```python
from build123d import *

# Parameters (mm, degrees)
SKETCH_1_W      = 33
SKETCH_1_H      = 22
EXTRUDE_1_DEPTH = 3


with BuildPart() as part:
    # 草图1 → 凸台-拉伸1 (new body)
    with BuildSketch(Plane.XY):
        Polygon((12.097999847, 68.896913641), (23.174949538, 68.896913641), (23.174949538, -21.103086359), (33.727403861, -21.103086359), (33.727403861, -81.103086359), (13.227403861, -81.103086359), (13.227403861, -107.603086359), (-25.772596139, -107.603086359), (-25.772596139, -81.103086359), (-46.272596139, -81.103086359), (-46.272596139, -21.103086359), (-36.272596139, -21.103086359), (-36.272596139, 68.896913641), (-25.195646449, 68.896913641), (-25.195646449, -21.103086359), (12.097999847, -21.103086359), align=None)
        with BuildLine():
            Line((-33.148823301, 45.73159086), (-33.148823301, 60.73159086))
            ThreePointArc((-33.148823301, 60.73159086), (-31.548823301, 62.33159086), (-29.948823301, 60.73159086))
            Line((-29.948823301, 60.73159086), (-29.948823301, 45.73159086))
            ThreePointArc((-29.948823301, 45.73159086), (-31.548823301, 44.13159086), (-33.148823301, 45.73159086))
        make_face(mode=Mode.SUBTRACT)
        with BuildLine():
            Line((20.051176699, 45.73159086), (20.051176699, 60.73159086))
            ThreePointArc((20.051176699, 60.73159086), (18.451176699, 62.33159086), (16.851176699, 60.73159086))
            Line((16.851176699, 60.73159086), (16.851176699, 45.73159086))
            ThreePointArc((16.851176699, 45.73159086), (18.451176699, 44.13159086), (20.051176699, 45.73159086))
        make_face(mode=Mode.SUBTRACT)
        with Locations((-6.272596139, -93.603086359)):
            Rectangle(SKETCH_1_W, SKETCH_1_H, mode=Mode.SUBTRACT)
    extrude(amount=EXTRUDE_1_DEPTH)


solid = part.part
```
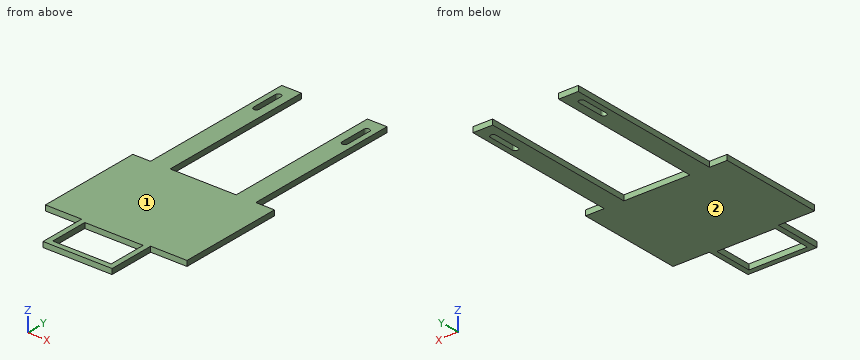
For this review, take the finished solid that the model builds, in its own axes (mm). Face numbers are marked on the shaded views. Round coordinates to 2 decimals unless told otherwise and drop trailing zeros. Write each loop counter-clockwise with the first axis right and the second up, starting at its lowest first coordinate (ties: lowest second). Pieces come first, ordered by that corner, then holes. Notation, with made-up numbers: (-21.75, -2) -> (26.25, -2) arc R8 ccw to (26.25, 8) -> close; hole circle Ø11 at (-31.75, 70.25). An arc over 180 degrees is marked (long way). One line per question, with ' | ' between items. Start each with the question number.
(1) For line 1 along Y through (x, z) = (-11.5, 2.15); line 2 along X through (y, z) = (4.5, 2.2); line 3 along X through (y, z) = (54.5, 2), list the stretches that pass through material, from the lowest coordinate up. Write a range as from..to.
(2) Add section B-B, the plane z = 0.7. Write out the cut boundary in (x, y), plus the area to 3 significant figures.
(3) Mouldability with a two-part tool opening along Z and no side actions: class the marked faces 1 and 2 as released by +Z, released by -Z, zero draft, split by the parting line, or undercut.
(4) Add section C-C, the plane x = 8. Write out the cut boundary in (y, z).
(5) Insertion check: P1, Ø0.9, axis at x = -39, z = 1, coming from the -Y side; P2, Ø0.9, axis at y = 51, z = 1, coming from the -X side; P3, Ø1.5, axis at x = -10, z = 1, coming from the +Y side. Each pin has a flat end and moves straight along its axis. Give the tip position at first contact, or say it passes through.
(6) Add section D-D, the plane x = -27.5. Write out the cut boundary in (y, z).
(7) Add section A-A, the plane y = 38. Write out the cut boundary in (x, z), plus the area to 3 significant figures.
Answer list:
1) line 1: -107.6..-104.6, -82.6..-21.1 | line 2: -36.27..-25.2, 12.1..23.17 | line 3: -36.27..-33.15, -29.95..-25.2, 12.1..16.85, 20.05..23.17
2) outline: (-46.27, -81.1) -> (-25.77, -81.1) -> (-25.77, -107.6) -> (13.23, -107.6) -> (13.23, -81.1) -> (33.73, -81.1) -> (33.73, -21.1) -> (23.17, -21.1) -> (23.17, 68.9) -> (12.1, 68.9) -> (12.1, -21.1) -> (-25.2, -21.1) -> (-25.2, 68.9) -> (-36.27, 68.9) -> (-36.27, -21.1) -> (-46.27, -21.1) -> close; hole (-33.15, 45.73) arc R1.6 ccw to (-29.95, 45.73) -> (-29.95, 60.73) arc R1.6 ccw to (-33.15, 60.73) -> close; hole (-22.77, -104.6) -> (10.23, -104.6) -> (10.23, -82.6) -> (-22.77, -82.6) -> close; hole (16.85, 45.73) arc R1.6 ccw to (20.05, 45.73) -> (20.05, 60.73) arc R1.6 ccw to (16.85, 60.73) -> close | area: 6,990 mm²
3) face 1: released by +Z | face 2: released by -Z
4) outline: (-107.6, 0) -> (-104.6, 0) -> (-104.6, 3) -> (-107.6, 3) -> close; (-82.6, 0) -> (-21.1, 0) -> (-21.1, 3) -> (-82.6, 3) -> close
5) P1: y = -81.1 | P2: x = -36.27 | P3: y = -21.1
6) outline: (-81.1, 0) -> (68.9, 0) -> (68.9, 3) -> (-81.1, 3) -> close
7) outline: (-36.27, 0) -> (-25.2, 0) -> (-25.2, 3) -> (-36.27, 3) -> close; (12.1, 0) -> (23.17, 0) -> (23.17, 3) -> (12.1, 3) -> close | area: 66.5 mm²
